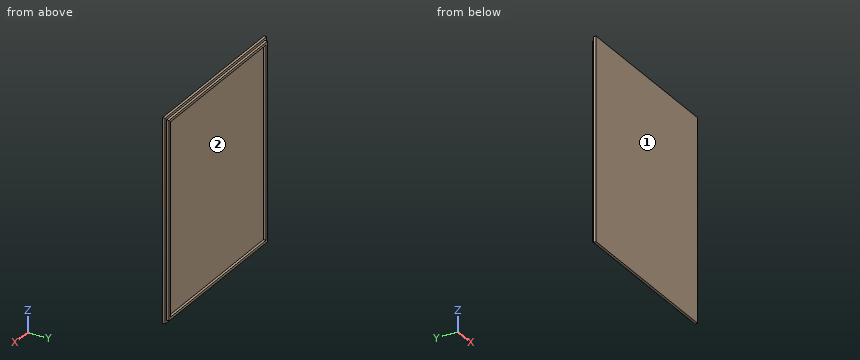
Autodesk Inventor part; units mm, degrees
ref_plane "YZ Plane" through (0, 0, 0) normal (1, 0, 0) x (0, 1, 0)
ref_plane "XZ Plane" through (0, 0, 0) normal (0, 1, 0) x (-1, 0, 0)
ref_plane "XY Plane" through (0, 0, 0) normal (0, 0, 1) x (1, 0, 0)
sketch "Sketch1" plane through (0, 0, 0) normal (0, 1, 0) x (-1, 0, 0)
  line L0 (0, 0) -> (-171.45, 0)
  line L1 (-171.45, 0) -> (-171.45, -203.2)
  line L2 (-171.45, -203.2) -> (0, -203.2)
  line L3 (0, -203.2) -> (0, 0)
  dimension "d0" = 171.45
  dimension "d2" = 203.2
extrude "Extrusion1" add sketch "Sketch1" against normal blind 2.54
sketch "Sketch4" plane through (0, -2.54, 0) normal (0, -1, 0) x (1, 0, 0)
  line L0 (168.91, -2.54) -> (2.54, -2.54)
  line L1 (2.54, -2.54) -> (2.54, -200.66)
  line L2 (2.54, -200.66) -> (168.91, -200.66)
  line L3 (168.91, -200.66) -> (168.91, -2.54)
  line L4 (171.45, 0) -> (171.45, -203.2)
  line L5 (171.45, -203.2) -> (0, -203.2)
  line L6 (0, 0) -> (171.45, 0)
  line L7 (0, -203.2) -> (0, 0)
  dimension "d20" = 2.54
  dimension "d21" = 2.54
  dimension "d22" = 2.54
  dimension "d23" = 2.54
extrude "Extrusion3" add sketch "Sketch4" against normal blind 5.08 contours L3 L2 L1 L0
sketch "Sketch6" plane through (0, 2.54, 0) normal (0, 1, 0) x (1, 0, 0)
  line L0 (5.08, 5.08) -> (166.37, 5.08)
  line L1 (166.37, 5.08) -> (166.37, 198.12)
  line L2 (166.37, 198.12) -> (5.08, 198.12)
  line L3 (5.08, 198.12) -> (5.08, 5.08)
  line L4 (2.54, 200.66) -> (2.54, 2.54)
  line L5 (168.91, 200.66) -> (2.54, 200.66)
  line L6 (168.91, 2.54) -> (168.91, 200.66)
  line L7 (2.54, 2.54) -> (168.91, 2.54)
  point P0 (0, 0)
  dimension "d24" = 2.54
  dimension "d25" = 2.54
  dimension "d26" = 2.54
  dimension "d27" = 2.54
extrude "Extrusion4" cut sketch "Sketch6" against normal blind 2.54 contours L3 L2 L1 L0
properties part number "Lid"
Verification items for the finished model (mm, model axes). Face numbers are marked on the shaded views. Round coordinates to 2 decimals unless told otherwise and drop trailing zeros. Order: outer loops, then holes, each group sorted by start corner. A loop starts at its lowest first (then second) coordinate and runs counter-clockwise, first axis right, second up. Notation, with made-up numbers: (53, -24) -> (95, -24) arc R21 ccw to (95, -5) -> close; hole circle Ø3 at (79.5, -23). An arc over 180 degrees is marked (long way). Put each result on its own line as item: value.
1) Section check B-B (z = -184.5). Record the cut outline in (x, y), then the cut area to 3 significant figures.
Final values:
outline: (0, -2.54) -> (171.45, -2.54) -> (171.45, 0) -> (168.91, 0) -> (168.91, 2.54) -> (166.37, 2.54) -> (166.37, 0) -> (5.08, 0) -> (5.08, 2.54) -> (2.54, 2.54) -> (2.54, 0) -> (0, 0) -> close
area: 448 mm^2
2) Mould release check, pull along Z, two halves, no side actions. Record for the marked faces 1 and 2: +Z half, -Z half, draft (parallel to the pull), parting line (faces both ways), or undercut.
Final values:
face 1: draft
face 2: undercut
3) Depth check by flat-ended pin: pin 1 (1.3 mm diameter, centred on x = 126.5, y = 2, fed in from -Z); pin 2 (2 mm diameter, centred on y = 1.5, z = -137.5, fed in from -X); pin 3 (2 mm diameter, centred on x = 101, y = 1.5, fed in from +Z). Enter the tip coordinate at first touch or a pass-through.
Final values:
pin 1: stops at z = -200.66
pin 2: stops at x = 2.54
pin 3: stops at z = -2.54
4) Material ranges on line 1 (X direction, y = 1.85, z = -144); line 2 (Z direction, x = 141, y = 1.65); line 3 (Y direction, x = 26, z = -135), recorded low to high.
Final values:
line 1: x = 2.54 to 5.08, 166.37 to 168.91
line 2: z = -200.66 to -198.12, -5.08 to -2.54
line 3: y = -2.54 to 0
5) Section check A-A (y = 1.7). Record the cut outline in (x, z), then the cut area to 3 significant figures.
Final values:
outline: (2.54, -200.66) -> (168.91, -200.66) -> (168.91, -2.54) -> (2.54, -2.54) -> close; hole (5.08, -198.12) -> (166.37, -198.12) -> (166.37, -5.08) -> (5.08, -5.08) -> close
area: 1,830 mm^2
6) Section check C-C (x = 155). Record the cut outline in (y, z).
Final values:
outline: (-2.54, -203.2) -> (0, -203.2) -> (0, -200.66) -> (2.54, -200.66) -> (2.54, -198.12) -> (0, -198.12) -> (0, -5.08) -> (2.54, -5.08) -> (2.54, -2.54) -> (0, -2.54) -> (0, 0) -> (-2.54, 0) -> close
